Geometry check sheet. Reference: the model listing, model coordinates, mm. A direction names the side the tool comes from. Coordinates: 2 decimals unless noted, no trailing zeros. Loops run counter-clockwise (first coordinate to the right, second up) from the corner with the lowest first, then second, coordinate; pieces in that order, holes last.
from build123d import *

# Parameters (mm, degrees)
F0_W     = 44.45
F0_H     = 12.7
F1_DEPTH = 12.7
F2_R     = 2.794
F3_DEPTH = 12.701
F4_R     = 2.794
F5_DEPTH = 12.701
F6_R     = 4.7625
F7_DEPTH = 5.08
F8_R     = 4.7625
F9_DEPTH = 5.08


with BuildPart() as f1:
    # F0 (on Top) → F1 (new body)
    with BuildSketch(Plane.XY):
        with Locations((0, -6.35)):
            Rectangle(F0_W, F0_H)
    extrude(amount=F1_DEPTH)

    # F2 (on face) → F3 (cut, through all)
    with BuildSketch(Plane.XY.offset(12.7)):
        with Locations((15.875, -6.35)):
            Circle(F2_R)
    extrude(amount=-F3_DEPTH, mode=Mode.SUBTRACT)

    # F4 (on face) → F5 (cut, through all)
    with BuildSketch(Plane(origin=(0, 0, 0), x_dir=(1, 0, 0), z_dir=(0, 0, -1))):
        with Locations((-15.875, 6.35)):
            Circle(F4_R)
    extrude(amount=-F5_DEPTH, mode=Mode.SUBTRACT)

    # F6 (on face) → F7 (cut)
    with BuildSketch(Plane.XY.offset(12.7)):
        with Locations((15.875, -6.35)):
            Circle(F6_R)
    extrude(amount=-F7_DEPTH, mode=Mode.SUBTRACT)

    # F8 (on face) → F9 (cut)
    with BuildSketch(Plane(origin=(0, 0, 0), x_dir=(1, 0, 0), z_dir=(0, 0, -1))):
        with Locations((-15.875, 6.35)):
            Circle(F8_R)
    extrude(amount=-F9_DEPTH, mode=Mode.SUBTRACT)


solid = f1.part
1) Material ranges on probe 1 along X at (y, z) = (-5.5, 11.5) (3 decimals); probe 2 along Z at (x, y) = (19, -4.25); probe 3 along X at (y, z) = (-3.5, 9) (3 decimals), recorded low to high.
Data:
probe 1: x = -22.225 to -18.537, -13.213 to 11.189, 20.561 to 22.225
probe 2: z = 0 to 7.62
probe 3: x = -22.225 to 12.059, 19.691 to 22.225
2) Section check A-A on y = -6.35. Record the cut outline in (x, z) (1 decimal).
Data:
outline: (-22.2, 0) - (-20.6, 0) - (-20.6, 5.1) - (-18.7, 5.1) - (-18.7, 12.7) - (-22.2, 12.7) - close; (-13.1, 5.1) - (-11.1, 5.1) - (-11.1, 0) - (13.1, 0) - (13.1, 7.6) - (11.1, 7.6) - (11.1, 12.7) - (-13.1, 12.7) - close; (18.7, 0) - (22.2, 0) - (22.2, 12.7) - (20.6, 12.7) - (20.6, 7.6) - (18.7, 7.6) - close
3) Access from +Z, -Z, +X, -X, +Y, -Y to the whole of each face (thin tool, end or side, straight path). Record for faces 5 (the flat face through (15.8, -9.5, 7.62)), 6 (the cylindrical face through (-13.21, -7.19, 8.84)), 7 (the cylindrical face through (-20.633, -6.559, 2.504)).
Data:
face 5: +Z
face 6: +Z, -Z
face 7: -Z
4) Section check D-D on y = -4. Record the cut outline in (x, z) (3 decimals).
Data:
outline: (-22.225, 0) - (-20.017, 0) - (-20.017, 5.08) - (-17.386, 5.08) - (-17.386, 12.7) - (-22.225, 12.7) - close; (-14.364, 5.08) - (-11.733, 5.08) - (-11.733, 0) - (14.364, 0) - (14.364, 7.62) - (11.733, 7.62) - (11.733, 12.7) - (-14.364, 12.7) - close; (17.386, 0) - (22.225, 0) - (22.225, 12.7) - (20.017, 12.7) - (20.017, 7.62) - (17.386, 7.62) - close
5) Mould release check, pull along Y, two halves, no side actions. Record for faces 1 (the flat face through (0, 0, 6)), 2 (the flat face through (0, -12.7, 6)), 3 (the flat face through (22.225, -6, 6)), 4 (the flat face through (-14, -4, 5.08)): +Y half, -Y half, draft (parallel to the pull), parting line (faces both ways), or undercut.
Data:
face 1: +Y half
face 2: -Y half
face 3: draft
face 4: undercut
6) Section check B-B on z = 11. Count the separate pieces of the cut face and the enclosed holes in it, and give its area (3 significant figures).
Data:
separate pieces: 1
enclosed holes: 2
area: 469 mm2
7) Depth check by flat-ended pin: pin 1 (7.5 mm diameter, centred on x = -15.875, y = -6.35, fed in from +Z); pin 2 (3 mm diameter, centred on x = 16, y = -4.5, fed in from +Z); pin 3 (5 mm diameter, centred on x = 15.875, y = -6.35, fed in from -Z); pin 4 (7.5 mm diameter, centred on x = -16, y = -5.5, fed in from -Z). Enter the tip coordinate at first touch or a pass-through.
Data:
pin 1: stops at z = 12.7
pin 2: stops at z = 7.62
pin 3: passes through
pin 4: stops at z = 5.08
8) Section check C-C on y = -2. Record the cut outline in (x, z) (3 decimals).
Data:
outline: (-22.225, 0) - (-17.814, 0) - (-17.814, 5.08) - (-13.936, 5.08) - (-13.936, 0) - (22.225, 0) - (22.225, 12.7) - (17.814, 12.7) - (17.814, 7.62) - (13.936, 7.62) - (13.936, 12.7) - (-22.225, 12.7) - close
